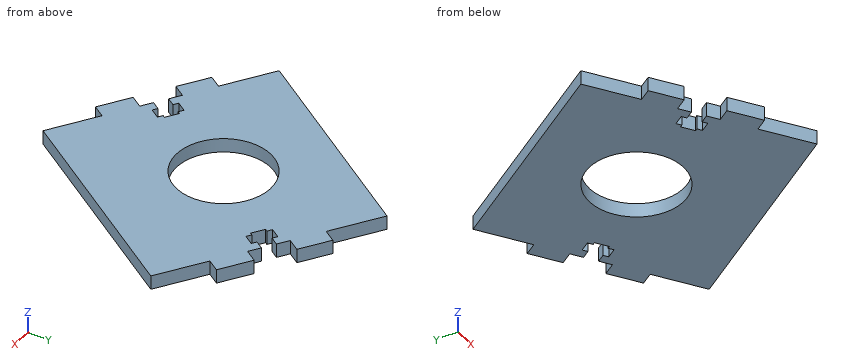
Autodesk Inventor part; units mm, degrees
ref_plane "YZ Plane" through (0, 0, 0) normal (1, 0, 0) x (0, 1, 0)
ref_plane "XZ Plane" through (0, 0, 0) normal (0, 1, 0) x (-1, 0, 0)
ref_plane "XY Plane" through (0, 0, 0) normal (0, 0, 1) x (1, 0, 0)
sketch "Sketch1" plane through (0, 0, 0) normal (0, 0, 1) x (1, 0, 0)
  circle A0 centre (11.8, 0) radius 10.15
  line L0 (0.848, -26.1294) -> (7.0019, -30.4166)
  line L1 (7.0019, -30.4166) -> (8.7168, -27.9551)
  line L2 (-11.9996, -17.1789) -> (-6.1263, -21.2706)
  line L3 (-6.1263, -21.2706) -> (-4.4115, -18.8091)
  line L4 (-4.4115, -18.8091) -> (-2.1551, -20.381)
  line L5 (-2.1551, -20.381) -> (-1.0118, -18.74)
  line L6 (-1.0118, -18.74) -> (-1.9554, -18.0826)
  line L7 (-1.9554, -18.0826) -> (-0.5835, -16.1134)
  line L8 (-0.5835, -16.1134) -> (0.3601, -16.7708)
  line L9 (0.3601, -16.7708) -> (0.7031, -16.2785)
  line L10 (0.7031, -16.2785) -> (3.1646, -17.9933)
  line L11 (3.1646, -17.9933) -> (2.8216, -18.4856)
  line L12 (2.8216, -18.4856) -> (3.7652, -19.143)
  line L13 (3.7652, -19.143) -> (2.3933, -21.1123)
  line L14 (2.3933, -21.1123) -> (1.4497, -20.4549)
  line L15 (1.4497, -20.4549) -> (0.3065, -22.0959)
  line L16 (0.3065, -22.0959) -> (2.5629, -23.6679)
  line L17 (2.5629, -23.6679) -> (0.848, -26.1294)
  line L18 (8.7168, -27.9551) -> (18.3578, -34.6717)
  line L19 (18.3578, -34.6717) -> (46.5961, 5.8617)
  line L20 (46.5961, 5.8617) -> (36.9551, 12.5783)
  line L21 (36.9551, 12.5783) -> (38.67, 15.0399)
  line L22 (38.67, 15.0399) -> (32.5161, 19.3271)
  line L23 (32.5161, 19.3271) -> (30.8012, 16.8655)
  line L24 (30.8012, 16.8655) -> (28.5448, 18.4375)
  line L25 (28.5448, 18.4375) -> (27.4015, 16.7965)
  line L26 (27.4015, 16.7965) -> (28.3451, 16.1391)
  line L27 (28.3451, 16.1391) -> (26.9732, 14.1699)
  line L28 (26.9732, 14.1699) -> (26.0296, 14.8272)
  line L29 (26.0296, 14.8272) -> (25.6867, 14.3349)
  line L30 (25.6867, 14.3349) -> (23.2251, 16.0498)
  line L31 (23.2251, 16.0498) -> (23.5681, 16.5421)
  line L32 (23.5681, 16.5421) -> (22.6245, 17.1995)
  line L33 (22.6245, 17.1995) -> (23.9964, 19.1687)
  line L34 (23.9964, 19.1687) -> (24.94, 18.5114)
  line L35 (24.94, 18.5114) -> (26.0833, 20.1524)
  line L36 (26.0833, 20.1524) -> (23.8268, 21.7244)
  line L37 (23.8268, 21.7244) -> (25.5417, 24.1859)
  line L38 (25.5417, 24.1859) -> (19.6685, 28.2776)
  line L39 (19.6685, 28.2776) -> (17.9536, 25.8161)
  line L40 (17.9536, 25.8161) -> (8.0319, 32.7281)
  line L41 (8.0319, 32.7281) -> (-20.2064, -7.8053)
  line L42 (-20.2064, -7.8053) -> (-10.2847, -14.7174)
  line L43 (-10.2847, -14.7174) -> (-11.9996, -17.1789)
  point P0 (0, 0)
extrude "Extrusion1" add sketch "Sketch1" along normal blind 3
Geometry check sheet. Reference: the model listing, model coordinates, mm. Coordinates: 2 decimals unless noted, no trailing zeros. Order: outer loops, then holes, each group sorted by start corner. A loop starts at its lowest first (then second) coordinate and runs counter-clockwise, first axis right, second up. Notation, with made-up numbers: (-6, 26.5) -> (34, 26.5) arc R15 cw to (34, 41.5) -> close; hole circle Ø7 at (5.25, 55.25). An arc over 180 degrees is marked (long way). Use a Markdown table: item, result. Add a question column.
1. Cross-section at A-A (y = 0). Enter the section's corners in (x, z), and give its area (3 significant figures).
2. Cross-section at C-C (x = 41.5). Enter the section's corners in (y, z).
3. Go/stop test with a flat-tipped pin: pin 1 Ø12 at (x, y) = (16, -4.5) entering from -Z. Record where the tip stops, or that it passes through.
4. Material ranges on L1, parallel to X at y = 14.5, z = 1.45; L2, parallel to Y at x = 24, z = 0.5; L3, parallel to Y at x = 0.5, z = 1.3, recorded low to high.
5. Cross-section at B-B (x = 11.8). Enter the section's corners in (y, z), and give its area (3 significant figures).
6. Cross-section at D-D (y = -12.5). Enter the section's corners in (x, z).
Filled sheet:
| question | item | result |
|---|---|---|
| 1 | outline | (-14.77, 0) -> (1.65, 0) -> (1.65, 3) -> (-14.77, 3) -> close; (21.95, 0) -> (42.51, 0) -> (42.51, 3) -> (21.95, 3) -> close |
| 1 | area | 111 mm2 |
| 2 | outline | (-1.45, 0) -> (9.41, 0) -> (9.41, 3) -> (-1.45, 3) -> close |
| 3 | pin 1 | z = 0 |
| 4 | L1 | -4.67 to 25.45, 25.8 to 26.5, 27.2 to 38.29 |
| 4 | L2 | -26.57 to 15.51, 19.17 to 21.6, 21.97 to 25.26 |
| 4 | L3 | -22.23 to -21.82, -16.57 to 21.92 |
| 5 | outline | (-30.1, 0) -> (-10.15, 0) -> (-10.15, 3) -> (-30.1, 3) -> close; (10.15, 0) -> (30.1, 0) -> (30.1, 3) -> (10.15, 3) -> close |
| 5 | area | 120 mm2 |
| 6 | outline | (-13.47, 0) -> (33.8, 0) -> (33.8, 3) -> (-13.47, 3) -> close |
